Geometry check sheet. Reference: the model listing, model coordinates, mm. A direction names the side the tool comes from. Round coordinates to 2 decimals unless told otherwise and drop trailing zeros. Write each loop counter-clockwise with the first axis right and the second up, starting at its lowest first coordinate (ties: lowest second). Pieces come first, ordered by that corner, then holes. Notation, with made-up numbers: M 73.25,7.5 L 93.25,7.5 A8 cw 93.25,11.5 Z; hole C 18.25,38 d8. An arc over 180 degrees is marked long. Use a Markdown table: item, result.
```python
from build123d import *

# Parameters (mm, degrees)
ESBO_O2_W                = 16
ESBO_O2_H                = 6
ESBO_O2_R                = 1
RESSALTO_EXTRUS_O4_DEPTH = 2.5
RESSALTO_EXTRUS_O6_DEPTH = 20


with BuildPart() as part:
    # Esboço2 → Ressalto-extrusão4 (new body)
    with BuildSketch(Plane(origin=(0, 0, 0), x_dir=(1, 0, 0), z_dir=(0, 1, 0))):
        Rectangle(ESBO_O2_W, ESBO_O2_H)
        with Locations(Location((-5.75, -1, 0), (0, 0, 270))):
            Circle(ESBO_O2_R, mode=Mode.SUBTRACT)
        with Locations(Location((5.75, -1, 0), (0, 0, 270))):
            Circle(ESBO_O2_R, mode=Mode.SUBTRACT)
    extrude(amount=RESSALTO_EXTRUS_O4_DEPTH)

    # Esboço4 → Ressalto-extrusão6 (add)
    with BuildSketch(Plane(origin=(0, 2.5, 0), x_dir=(1, 0, 0), z_dir=(0, 1, 0))):
        with BuildLine():
            Line((13.2, 2.45), (-13.2, 2.45))
            Line((-13.2, 2.45), (-13.2, 9.55))
            Line((-13.2, 9.55), (-2.43874968, 9.55))
            ThreePointArc((-2.43874968, 9.55), (0, 6.5), (2.43874968, 9.55))
            Line((2.43874968, 9.55), (13.2, 9.55))
            Line((13.2, 9.55), (13.2, 2.45))
        make_face()
        with BuildLine():
            Line((3.290516677, 8.75), (12.4, 8.75))
            Line((12.4, 8.75), (12.4, 3.25))
            Line((12.4, 3.25), (0.4, 3.25))
            Line((0.4, 3.25), (0.4, 5.724332129))
            ThreePointArc((0.4, 5.724332129), (2.386135967, 6.720448476), (3.290516677, 8.75))
        make_face(mode=Mode.SUBTRACT)
        with BuildLine():
            Line((-0.4, 3.25), (-12.4, 3.25))
            Line((-12.4, 3.25), (-12.4, 8.75))
            Line((-12.4, 8.75), (-3.290516677, 8.75))
            ThreePointArc((-3.290516677, 8.75), (-2.386135967, 6.720448476), (-0.4, 5.724332129))
            Line((-0.4, 5.724332129), (-0.4, 3.25))
        make_face(mode=Mode.SUBTRACT)
    extrude(amount=-RESSALTO_EXTRUS_O6_DEPTH)


solid = part.part
```
Item 1: Cross-section at A-A, the plane z = 1. Record the cut outline in (x, y), and give its area (3 significant figures).
Outcome:
| item | result |
|---|---|
| outline | M -8,0 L -6.75,0 L -6.75,2.5 L -8,2.5 Z; M -4.75,0 L 4.75,0 L 4.75,2.5 L -4.75,2.5 Z; M 6.75,0 L 8,0 L 8,2.5 L 6.75,2.5 Z |
| area | 30.0 mm2 |
Item 2: Mould release check, pull along X, two halves, no side actions. Record for faces 4 (the face through (-8, 1, 0)), 5 (the face through (-8, -7, -8.75)), 6 (the face through (8, -7, -9.55)): +X half, -X half, draft (parallel to the pull), parting line (faces both ways), or undercut.
Outcome:
| item | result |
|---|---|
| face 4 | -X half |
| face 5 | undercut |
| face 6 | draft |
Item 3: Go/stop test with flat-tipped pins: pin 1 (2.5 mm diameter, centred on x = 2.5, z = -0.5, fed in from -Y); pin 2 (2.5 mm diameter, centred on x = -6.5, y = -6.5, fed in from +Z); pin 3 (3 mm diameter, centred on y = 1, z = 0.5, fed in from -X); pin 4 (5 mm diameter, centred on x = 9, z = -0.5, fed in from +Y). Record where each tip stops, or that it passes through.
Outcome:
| item | result |
|---|---|
| pin 1 | stops at y = 0 |
| pin 2 | stops at z = -2.45 |
| pin 3 | stops at x = -8 |
| pin 4 | stops at y = 2.5 |
Item 4: Cross-section at C-C, the plane x = 10.75. Record the cut outline in (y, z).
Outcome:
| item | result |
|---|---|
| outline | M -17.5,-9.55 L 2.5,-9.55 L 2.5,-8.75 L -17.5,-8.75 Z; M -17.5,-3.25 L 2.5,-3.25 L 2.5,-2.45 L -17.5,-2.45 Z |
Item 5: Access from +Z, -Z, +X, -X, +Y, -Y to the whole of each face (thin tool, end or side, straight path). Record for faces 1 (the face through (-8, -7, -9.55)), 2 (the face through (-6, -7, -3.25)), 3 (the face through (0, 0, 0)).
Outcome:
| item | result |
|---|---|
| face 1 | -Z, +X, -X, +Y, -Y |
| face 2 | +Y, -Y |
| face 3 | +Z, +X, -X, -Y |
Item 6: Cross-section at B-B, the plane y = 1. Record the cut outline in (x, z).
Outcome:
| item | result |
|---|---|
| outline | M -13.2,-9.55 L -2.44,-9.55 A2.5 cw long 2.44,-9.55 L 13.2,-9.55 L 13.2,-2.45 L 8,-2.45 L 8,3 L -8,3 L -8,-2.45 L -13.2,-2.45 Z; hole M -12.4,-8.75 L -3.29,-8.75 A3.3 cw -0.4,-5.72 L -0.4,-3.25 L -12.4,-3.25 Z; hole C -5.75,1 d2; hole M 0.4,-5.72 A3.3 cw 3.29,-8.75 L 12.4,-8.75 L 12.4,-3.25 L 0.4,-3.25 Z; hole C 5.75,1 d2 |
Item 7: Material ranges on line 1 along X through (y, z) = (1.45, 1); line 2 along X through (y, z) = (-5, -5.5); line 3 along X through (y, z) = (-3, -9), recorded low to high. Write a range as from..to.
Outcome:
| item | result |
|---|---|
| line 1 | x = -8..-6.75, -4.75..4.75, 6.75..8 |
| line 2 | x = -13.2..-12.4, -0.4..0.4, 12.4..13.2 |
| line 3 | x = -13.2..-2.5, 2.5..13.2 |
Item 8: Cross-section at D-D, the plane x = -5.75. Record the cut outline in (y, z).
Outcome:
| item | result |
|---|---|
| outline | M -17.5,-9.55 L 2.5,-9.55 L 2.5,-8.75 L -17.5,-8.75 Z; M -17.5,-3.25 L 2.5,-3.25 L 2.5,0 L 0,0 L 0,-2.45 L -17.5,-2.45 Z; M 0,2 L 2.5,2 L 2.5,3 L 0,3 Z |
